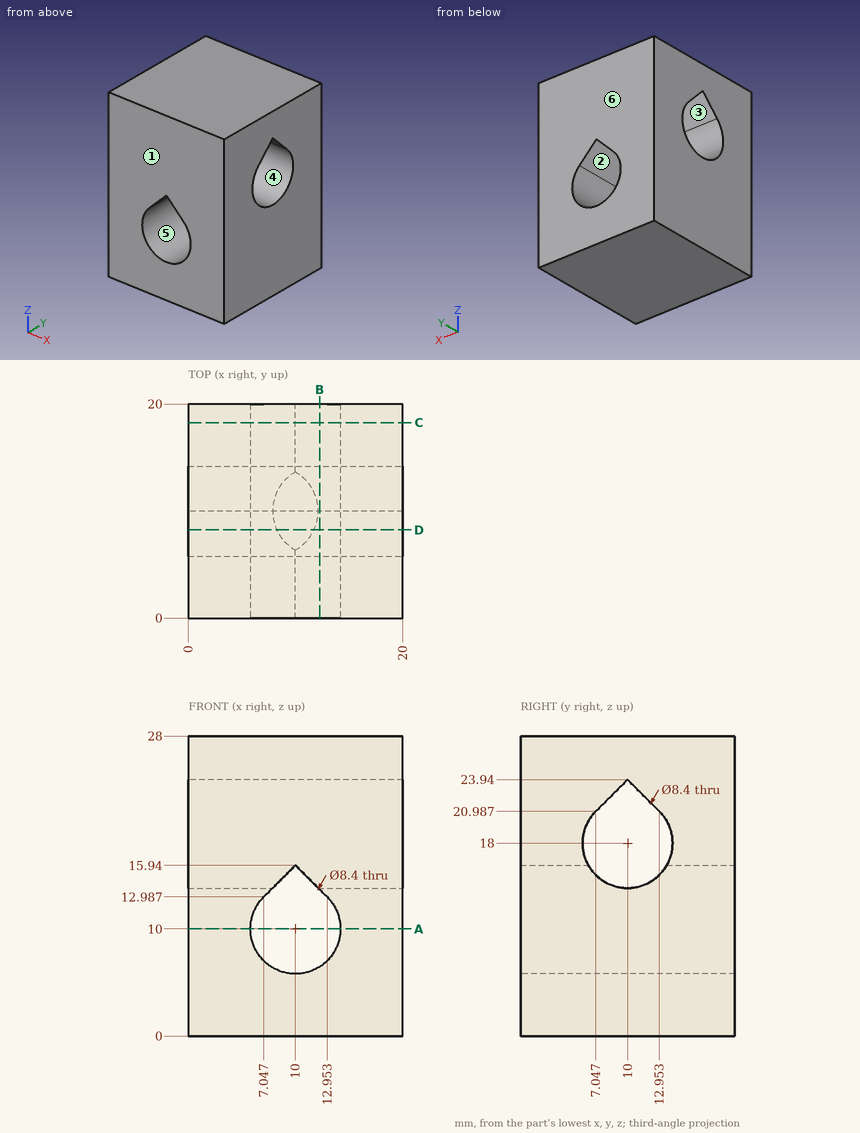
Design review of the part shown in the three views and the two pictorial views. Dimensions are in mm from the part's minimum x, y and z. A direction names the side the tool comes from. Give positions to 0.01 mm unless a question says otherwise; leave off trailing zeros. Loops run counter-clockwise (first coordinate to the right, second up) from the corner with the lowest first, then second, coordinate; pieces in that order, holes last. Notation, with made-up numbers: (41, -34) -> (49, -34) arc R15 ccw to (49, -20) -> close; hole circle Ø3 at (79, 81.25). An arc over 180 degrees is marked (long way). Write each question's results on one line, items separated by ' | '.
Q1. Take a section at D-D, the plane y = 8.25. Write out the cut boundary in (x, z), plus the area to 3 significant figures.
Reply:
outline: (0, 0) -> (20, 0) -> (20, 14.18) -> (11.76, 14.18) -> (12.95, 12.99) arc R4.2 cw (long way) to (7.05, 12.99) -> (8.24, 14.18) -> (0, 14.18) -> close; (0, 22.19) -> (20, 22.19) -> (20, 28) -> (0, 28) -> close | area: 344 mm²
Q2. Machinability: for the marked faces 1, 2 and 3, which of the approach directions +Z, -Z, +X, -X, +Y, -Y give a long, thin tool a straight path to every point of the face, cutting with its end or side? Answer none if there is none.
Reply:
face 1: +Z, -Z, +X, -X, -Y | face 2: +Y, -Y | face 3: +X, -X
Q3. Take a section at A-A, the plane z = 10. Write out the cut boundary in (x, y), plus the area to 3 significant figures.
Reply:
outline: (0, 0) -> (5.8, 0) -> (5.8, 20) -> (0, 20) -> close; (14.2, 0) -> (20, 0) -> (20, 20) -> (14.2, 20) -> close | area: 232 mm²
Q4. The part is to be moulded in two halves that separate along Y. For the marked faces 4, 5 and 6, say which applies: +Y half, -Y half, draft (parallel to the pull), parting line (faces both ways), or undercut.
Reply:
face 4: undercut | face 5: draft | face 6: +Y half
Q5. Take a section at B-B, the plane x = 12.25. Write out the cut boundary in (y, z), plus the area to 3 significant figures.
Reply:
outline: (0, 0) -> (20, 0) -> (20, 6.45) -> (0, 6.45) -> close; (0, 13.69) -> (20, 13.69) -> (20, 28) -> (0, 28) -> close; hole (7.05, 20.99) arc R4.2 ccw (long way) to (12.95, 20.99) -> (10, 23.94) -> close | area: 356 mm²
Q6. Take a section at C-C, the plane y = 18.25. Write out the cut boundary in (x, z), plus the area to 3 significant figures.
Reply:
outline: (0, 0) -> (20, 0) -> (20, 28) -> (0, 28) -> close; hole (7.05, 12.99) arc R4.2 ccw (long way) to (12.95, 12.99) -> (10, 15.94) -> close | area: 501 mm²
Q7. Wall thickness on L1, parallel to Z at x = 6.25, y = 6.5; L2, parallel to Y at x = 10, z = 19; L3, parallel to Z at x = 13.75, y = 15.25: over which ranges is each line inside the solid? List them lowest first.
Reply:
L1: z = 0 to 8.11, 11.89 to 15.68, 20.32 to 28 | L2: y = 0 to 5.92, 14.08 to 20 | L3: z = 0 to 8.11, 11.89 to 28
